For this review, take the finished solid that the model builds, in its own axes (mm). A direction names the side the tool comes from. Give positions to 0.01 mm unless a question says otherwise; leave off trailing zeros. Order: outer loops, then holes, each group sorted by start corner. A loop starts at its lowest first (then second) coordinate and runs counter-clockwise, first axis right, second up. Notation, with made-up numbers: (44.5, -2.75) -> (64.5, -2.75) arc R31 cw to (64.5, 31.25) -> close; hole circle Ø11 at (-25, -6). An arc over 180 degrees is marked (long way). One line per item, written item: value. Start each with the question number.
Autodesk Inventor part; units mm, degrees
ref_plane "XZ Plane" through (0, 0, 0) normal (0, 1, 0) x (-1, 0, 0)
ref_plane "XY Plane" through (0, 0, 0) normal (0, 0, 1) x (1, 0, 0)
sketch "スケッチ1" plane through (0, 0, 0) normal (0, 1, 0) x (-1, 0, 0)
  circle A0 centre (0, 0) radius 15
  dimension "d0" = 30
extrude "押し出し1" add sketch "スケッチ1" along normal blind 3
sketch "スケッチ2" plane through (0, 3, 0) normal (0, 1, 0) x (1, 0, 0)
  circle A0 centre (0, 0) radius 15
  line L0 (14.7817, -2.55) -> (8, -2.55)
  line L1 (8, -2.55) -> (8, -4.55)
  line L2 (8, 4.55) -> (8, 2.55)
  line L3 (-21, 0) -> (21, 0)
  line L4 (0, 21) -> (0, -21)
  line L5 (8, -4.55) -> (14.2933, -4.55)
  line L6 (14.7817, -2.55) -> (14.2933, -4.55)
  line L7 (8, 2.55) -> (14.7817, 2.55)
  line L8 (8, 2.55) -> (14.7817, 2.55) construction
  line L9 (8, 4.55) -> (14.2933, 4.55)
  line L10 (14.7817, 2.55) -> (14.2933, 4.55)
  point P0 (11.3908, -2.55)
  point P1 (8, -3.55)
  point P2 (8, 3.55)
  dimension "d16" = 2
  dimension "d27" = 8
  dimension "d28" = 2.55
  dimension "d29" = 8
  dimension "d31" = 2
  dimension "d33" = 2.55
extrude "押し出し2" add sketch "スケッチ2" along normal blind 11 contours L7 L2 L9 L10 | L6 L5 L1 L0
sketch "スケッチ4" plane through (14.2933, 3, -4.55) normal (0, 0, -1) x (-1, 0, 0)
  circle A0 centre (2.5, 8) radius 1.3
  line L0 (29.2933, 0) -> (0, 0)
  line L1 (6.2933, 0) -> (6.2933, 11)
  line L2 (0, 0) -> (0, 11)
  point P0 (14.2933, -3)
  dimension "d34" = 2.6
  dimension "d35" = 8
  dimension "d42" = 2.5
extrude "押し出し4" cut sketch "スケッチ4" against normal through all
sketch "スケッチ5" plane through (0, 3, 0) normal (0, 1, 0) x (1, 0, 0)
  circle A0 centre (0, 0) radius 4
  dimension "d39" = 8
extrude "押し出し5" add sketch "スケッチ5" along normal blind 11
sketch "スケッチ6" plane through (0, 0, 0) normal (1, 0, 0) x (0, 1, 0)
  line L0 (3, -4.55) -> (3, 4.55)
  line L1 (3, -2.55) -> (3, -4.55)
  line L2 (3, 2.55) -> (3, -2.55)
  line L3 (3, 4.55) -> (3, 2.55)
  line L4 (0, -15) -> (0, 15)
  line L5 (0, -15) -> (3, -15)
  point P0 (0, 0)
  point P1 (13, 0)
  dimension "d43" = 15
  dimension "d44" = 10
ref_plane "作業平面1" through (0, 13, 0) normal (0, -0.1736, 0.9848) x (1, 0, 0)
sketch "スケッチ7" plane through (0, 13, 0) normal (0, -0.1736, 0.9848) x (1, 0, 0)
  line L0 (1.5, -3) -> (-1.5, -3)
  line L1 (1.5, -3) -> (1.5, -3.5)
  line L2 (1.5, -3.5) -> (-1.5, -3.5)
  line L3 (-1.5, -3.5) -> (-1.5, -3)
  line L4 (0, -19.2066) -> (0, 7.3889)
  line L5 (-21, 0) -> (21, 0)
  point P0 (0, -12.8025)
  point P1 (1.5, -3.25)
  dimension "d46" = 3
  dimension "d47" = 0.5
  dimension "d48" = 1.5
  dimension "d49" = 3
extrude "押し出し6" cut sketch "スケッチ7" along normal blind 10
pattern_circular "円形状パターン1" count 4 over 360 about axis through (0, 3, 0) along (0, 1, 0) of "押し出し6"
properties part number "exp_latch_base_rev0"
Q1. For line 1 along Z through (x, y) = (8.75, 13.25); line 2 along Y through (x, z) = (-12, 2.5); line 3 along X through (y, z) = (2.5, -7.75), list the stretches that pass through material, from the lowest coordinate up.
Q2. Take a section at C-C (z = -9). State the section outline as (x, y) points.
Q3. Mouldability with a two-part tool opening along Z and no side actions: class faces 1 (the flat face through (14.54, 8.42, 3.54)), 2 (the flat face through (-2.732, 9.472, 0.021)), 3 (the flat face through (11, 14, -4)) as pulls with the +Z half, pulls with the -Z half, needs draft (parallel to the pull), parting line crosses it, or undercut.
Q4. Take a section at B-B (x = 12). State the section outline as (y, z) points.
Q5. Take a section at A-A (y = 4). State the section outline as (x, z) points, and give its area (3 significant figures).
Q6. Take a section at D-D (x = -7.25). State the section outline as (y, z) points, and give its area (3 significant figures).
Q7. For faces 4 (the flat face through (11, 8, 2.55)), 5 (the flat face through (1.5, 9.2, 2.6)), 6 (the cylindrical face through (11.96, 12.29, 3.54)), list the 3-axis set-ups (+Z, -Z, +X, -X, +Y, -Y) from which the entire face can be reached by the end or side of a thin tool; tool diameter is ignored.
Q8. For pin 1 Ø7.5 at (x, y) = (12, 10.5) entering from +Z; pin 2 Ø0.7 at (x, y) = (-2, 9.5) entering from -Z; pin 3 Ø6 at (x, y) = (1, 7) entering from -Z, all flat-tipped, find the tip position at first contact; note any pin that passes through.
Answers below:
1. line 1: z = -4.55 to -2.55, 2.55 to 4.55
1. line 2: y = 0 to 3
1. line 3: x = -12.84 to 12.84
2. outline: (-12, 0) -> (12, 0) -> (12, 3) -> (-12, 3) -> close
3. face 1: pulls with the +Z half
3. face 2: undercut
3. face 3: needs draft
4. outline: (0, -9) -> (3, -9) -> (3, -4.55) -> (9.72, -4.55) -> (9.72, -2.55) -> (3, -2.55) -> (3, 2.55) -> (9.72, 2.55) -> (9.72, 4.55) -> (3, 4.55) -> (3, 9) -> (0, 9) -> close; (12.28, -4.55) -> (14, -4.55) -> (14, -2.55) -> (12.28, -2.55) -> close; (12.28, 2.55) -> (14, 2.55) -> (14, 4.55) -> (12.28, 4.55) -> close
5. outline: circle Ø8 at (0, 0); (8, -4.55) -> (14.29, -4.55) -> (14.78, -2.55) -> (8, -2.55) -> close; (8, 2.55) -> (14.78, 2.55) -> (14.29, 4.55) -> (8, 4.55) -> close
5. area: 76.4 mm²
6. outline: (0, -13.13) -> (3, -13.13) -> (3, 13.13) -> (0, 13.13) -> close
6. area: 78.8 mm²
7. face 4: +X, +Y
7. face 5: none
7. face 6: +Z, -Z
8. pin 1: stops at z = 4.55
8. pin 2: stops at z = -3.64
8. pin 3: stops at z = -4
